```python
from build123d import *

# Parameters (mm, degrees)
F1_DEPTH = 38.1
F3_DEPTH = 12.7


with BuildPart() as f1:
    # F0 (on Front) → F1 (new body)
    with BuildSketch(Plane.XZ):
        Polygon((38.1, 0), (0, 0), (0, -38.1), (38.1, -38.1), (38.1, -25.4), (69.85, -25.4), (69.85, -12.7), (38.1, -12.7), align=None)
    extrude(amount=-F1_DEPTH)

    # F2 (on face) → F3 (join, through all)
    with BuildSketch(Plane.XY.offset(-12.7)):
        with BuildLine():
            Line((69.85, 38.1), (69.85, 0))
            ThreePointArc((69.85, 0), (88.9, 19.05), (69.85, 38.1))
        make_face()
    extrude(amount=-F3_DEPTH)


solid = f1.part
```
Can you work these out from the model? Positions are in its coordinate system, mm. A direction names the side the tool comes from. Coordinates: 2 decimals unless noted, no trailing zeros. Loops run counter-clockwise (first coordinate to the right, second up) from the corner with the lowest first, then second, coordinate; pieces in that order, holes last. Notation, with made-up numbers: (16, 2.25) - (65, 2.25) arc R16 cw to (65, 15.25) - close; hole circle Ø3 at (50, -25). An arc over 180 degrees is marked (long way). Answer as CSV lines item,"result". Start each with the question number.
1) Suppose I cut it at D-D (y = 32.5). Please give me the cut outline in (x, z).
2) Suppose I cut it at A-A (y = 19.05). Please give me the cut outline in (x, z).
3) Which directions (+Z, -Z, +X, -X, +Y, -Y) give clear straight access to the entire face, cutting with the end or side of a thin tool? Please do faces 1 (the flat face through (38.1, 19, -6)), 2 (the flat face through (27, 0, -19)), 3 (the flat face through (63, 19, -25.4)).
4) Suppose I cut it at C-C (z = -33). Please give me the cut outline in (x, y).
5) For pin 1 (11.5 mm diameter, centred on x = 70.5, y = 21.5, fed in from +Z); pin 2 (19 mm diameter, centred on x = 69, y = 18, fed in from -Z); pin 3 (3 mm diameter, centred on y = 7, z = -19, fed in from +X); pin 4 (3 mm diameter, centred on x = 40, z = -7, fed in from +Y), each with a flat end and sliding along its axis, tell me the tip position at first contact or that it passes through.
6) I need wall thicknesses on line 1 (Z direction, x = 58, y = 15.5); line 2 (X direction, y = 6, z = -29). Which ranges of each line are inside material? Lowest first, please. Write a range as from..to.
7) Suppose I cut it at B-B (x = 41). Please give me the cut outline in (y, z).
Check result:
1,outline,"(0, -38.1) - (38.1, -38.1) - (38.1, -25.4) - (83.34, -25.4) - (83.34, -12.7) - (38.1, -12.7) - (38.1, 0) - (0, 0) - close"
2,outline,"(0, -38.1) - (38.1, -38.1) - (38.1, -25.4) - (88.9, -25.4) - (88.9, -12.7) - (38.1, -12.7) - (38.1, 0) - (0, 0) - close"
3,face 1,"+Z, +X, +Y, -Y"
3,face 2,"+Z, -Z, +X, -X, -Y"
3,face 3,"-Z, +X, +Y, -Y"
4,outline,"(0, 0) - (38.1, 0) - (38.1, 38.1) - (0, 38.1) - close"
5,pin 1,"stops at z = -12.7"
5,pin 2,"stops at z = -25.4"
5,pin 3,"stops at x = 85.71"
5,pin 4,"passes through"
6,line 1,"z = -25.4..-12.7"
6,line 2,"x = 0..38.1"
7,outline,"(0, -25.4) - (38.1, -25.4) - (38.1, -12.7) - (0, -12.7) - close"
